CAD build for the part. Positions are in the model's coordinates, mm. Face numbers are marked on the shaded views. A direction names the side the tool comes from. Give positions to 0.01 mm unless a question says otherwise; leave off trailing zeros. Loops run counter-clockwise (first coordinate to the right, second up) from the corner with the lowest first, then second, coordinate; pieces in that order, holes last.
Item 1: Saw through at A-A on z = 5.25. Give the cut face in (x, y).
Item 2: Probe probe 1 along X at (y, z) = (5, 1); probe 2 along Z at (x, y) = (-3, 2.25); probe 3 along X at (y, z) = (0.5, 2). List the from-to ranges inside material, lowest first.
Item 3: Which spindle directions (+Z, -Z, +X, -X, +Y, -Y) get a long thin tool onto all of the face, cutting with end or side? Do the marked faces 1, 2 and 3. Say none if no direction does.
Item 4: Mould opens along Y. For the marked faces 4, 5, 6 and 7 say: released by +Y, released by -Y, zero draft, split by the parting line, or undercut.
Item 5: Saw through at D-D on z = 4.25. Give the cut face in (x, y), plus the area to 3 significant figures.
Item 6: Drop flat-ended pins along their axis: P1, Ø1, axis at y = 0.5, z = 2.5, coming from the +X side; P2, Ø0.6, axis at x = -5, z = 1, coming from the +Y side; P3, Ø2, axis at x = 0.5, y = 6.5, coming from the +Z side; P4, Ø5, axis at x = -4, y = 5.5, coming from the +Z side. Give the stop position or say it passes through.
from build123d import *

# Parameters (mm, degrees)
F1_DEPTH        = 1
F1_COPIES_COUNT = 6
F2_DEPTH        = 0.25
F2_COPIES_COUNT = 6
F3_R            = 9
F4_DEPTH        = 2
F5_R            = 1.99999


# Not quite as in the source:
# - a fillet or chamfer is up to 0.001 mm smaller than in the source, because OpenCascade refuses the exact size
# - a pattern or mirror of a feature is missing from the dataset's text; its kind, count and spacing are read off the source's solid


with BuildPart() as f1:
    # F0 (on Front) → F1 (new body, symmetric)
    with BuildSketch(Plane.XZ):
        with BuildLine():
            Line((6, 3), (6, 0))
            Line((6, 0), (7, 0))
            Line((7, 0), (7.8323762036, 3.1064702829))
            ThreePointArc((7.8323762036, 3.1064702829), (7.8578952387, 3.4958155202), (7.7324757811, 3.865289328))
            Line((7.7324757811, 3.865289328), (6.5, 6))
            Line((6.5, 6), (6, 6))
            Line((6, 6), (6, 3))
        make_face()
    extrude(amount=F1_DEPTH, both=True)


with BuildPart() as f1_copies_1:
    # F1_copies: instance of F1
    add(f1.part.rotate(Axis((0, 0, 0), (0, 0, 1)), 1 * 360 / F1_COPIES_COUNT))


with BuildPart() as f1_copies_2:
    # F1_copies: instance of F1
    add(f1.part.rotate(Axis((0, 0, 0), (0, 0, 1)), 2 * 360 / F1_COPIES_COUNT))


with BuildPart() as f1_copies_3:
    # F1_copies: instance of F1
    add(f1.part.rotate(Axis((0, 0, 0), (0, 0, 1)), 3 * 360 / F1_COPIES_COUNT))


with BuildPart() as f1_copies_4:
    # F1_copies: instance of F1
    add(f1.part.rotate(Axis((0, 0, 0), (0, 0, 1)), 4 * 360 / F1_COPIES_COUNT))


with BuildPart() as f1_copies_5:
    # F1_copies: instance of F1
    add(f1.part.rotate(Axis((0, 0, 0), (0, 0, 1)), 5 * 360 / F1_COPIES_COUNT))


with BuildPart() as f1_1:
    add(f1.part)

    # F0 (on Front) → F2 (join, symmetric)
    with BuildSketch(Plane.XZ):
        Polygon((6, 3), (4, 0), (6, 0), align=None)
    f2 = extrude(amount=F2_DEPTH, both=True)

    # F2_copies: F2 ×6 about axis
    f2_copies_axis = Axis((0, 0, 0), (0, 0, 1))
    for i in range(1, F2_COPIES_COUNT):
        add(f2.rotate(f2_copies_axis, i * 360 / F2_COPIES_COUNT))

    add(f1_copies_1.part)  # F4 merges F1_copies_1

    add(f1_copies_2.part)  # F4 merges F1_copies_2

    add(f1_copies_3.part)  # F4 merges F1_copies_3

    add(f1_copies_4.part)  # F4 merges F1_copies_4

    add(f1_copies_5.part)  # F4 merges F1_copies_5
    # F3 (on Top) → F4 (join)
    with BuildSketch(Plane.XY):
        Circle(F3_R)
    extrude(amount=-F4_DEPTH)

    # F5 (radius 2 in the source; OpenCascade refuses exactly that, so slightly less here)
    f5_edges = [f1_1.edges().sort_by_distance(p)[0] for p in [
        (-9, 0, -2),
    ]]
    fillet(f5_edges, radius=F5_R)


solid = f1_1.part
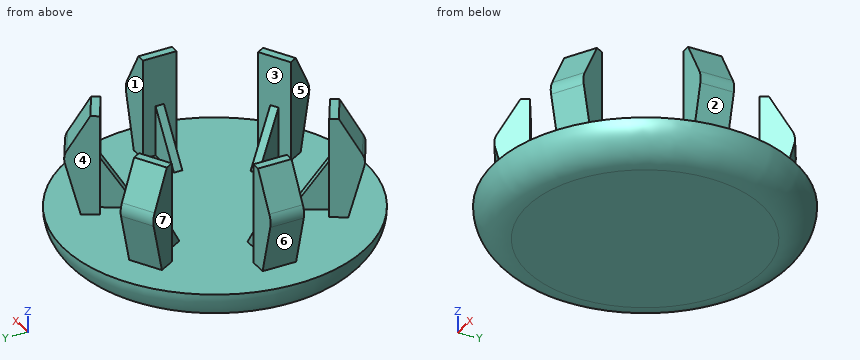
Results below:
1. outline: (-6.93, -1) - (-6, -1) - (-6, 1) - (-6.93, 1) - close; (-4.33, -5.5) - (-2.6, -6.5) - (-2.13, -5.7) - (-3.87, -4.7) - close; (-4.33, 5.5) - (-3.87, 4.7) - (-2.13, 5.7) - (-2.6, 6.5) - close; (2.13, -5.7) - (2.6, -6.5) - (4.33, -5.5) - (3.87, -4.7) - close; (2.13, 5.7) - (3.87, 4.7) - (4.33, 5.5) - (2.6, 6.5) - close; (6, -1) - (6.93, -1) - (6.93, 1) - (6, 1) - close
2. probe 1: x = -4.04 to -3.34, -3.18 to -2.6, 2.6 to 3.18, 3.34 to 4.04
2. probe 2: z = -2 to 0
2. probe 3: x = -7.54 to -6, 6 to 7.54
3. face 1: +Z, +X, -X, +Y
3. face 2: +X, +Y, -Y
3. face 3: +Z
4. face 4: released by +Y
4. face 5: released by -Y
4. face 6: zero draft
4. face 7: undercut
5. outline: (-7.51, -1) - (-6, -1) - (-6, 1) - (-7.51, 1) - close; (-4.62, -6) - (-2.89, -7) - (-2.13, -5.7) - (-3.87, -4.7) - close; (-4.62, 6) - (-3.87, 4.7) - (-2.13, 5.7) - (-2.89, 7) - close; (2.13, -5.7) - (2.89, -7) - (4.62, -6) - (3.87, -4.7) - close; (2.13, 5.7) - (3.87, 4.7) - (4.62, 6) - (2.89, 7) - close; (6, -1) - (7.51, -1) - (7.51, 1) - (6, 1) - close
5. area: 18.1 mm2
6. P1: stops at x = 7.8
6. P2: stops at y = 0.25
6. P3: stops at z = 0
6. P4: stops at z = 6
